```python
from build123d import *

# Parameters (mm, degrees)
SKETCH1_R           = 45
BOSS_EXTRUDE1_DEPTH = 600
SKETCH2_R           = 38.423285368
CUT_EXTRUDE1_DEPTH  = 604.365560834
CHAMFER1_SIZE       = 5.219704
CHAMFER1_SIZE_2     = 9.040792


with BuildPart() as part:
    # Sketch1 → Boss-Extrude1 (new body)
    with BuildSketch(Plane(origin=(0, 0, 0), x_dir=(1, 0, 0), z_dir=(0, 1, 0))):
        with Locations(Location((0, 0, 0), (0, 0, 270))):
            Circle(SKETCH1_R)
    extrude(amount=BOSS_EXTRUDE1_DEPTH)

    # Sketch2 → Cut-Extrude1 (cut, through all)
    with BuildSketch(Plane(origin=(0, 0, 0), x_dir=(1, 0, 0), z_dir=(0, 1, 0))):
        with Locations(Location((0, 0, 0), (0, 0, 270))):
            Circle(SKETCH2_R)
    extrude(amount=CUT_EXTRUDE1_DEPTH, mode=Mode.SUBTRACT)

    # Chamfer1
    # the kernel refuses this chamfer: 9.040792, 5.219704 mm, written as the material it takes off along each edge
    with BuildSketch(Plane(origin=(0, 600, 0), x_dir=(0, 0, 1), z_dir=(-1, 0, 0))) as chamfer1_piece_1:
        Polygon((45, -CHAMFER1_SIZE), (45 - CHAMFER1_SIZE_2, 0), (45, 0), align=None)
    revolve(axis=Axis((0, 600, 0), (0, 1, 0)), mode=Mode.SUBTRACT)
    with BuildSketch(Plane(origin=(0, 0, 0), x_dir=(0, 0, 1), z_dir=(-1, 0, 0))) as chamfer1_piece_2:
        Polygon((45, CHAMFER1_SIZE_2), (45 - CHAMFER1_SIZE, 0), (45, 0), align=None)
    revolve(axis=Axis((0, 0, 0), (0, 1, 0)), mode=Mode.SUBTRACT)


solid = part.part
```
The listing builds one solid part. Answer for the finished solid, in the listing's coordinates (mm). Round coordinates to 2 decimals unless told otherwise and drop trailing zeros. Order: outer loops, then holes, each group sorted by start corner. A loop starts at its lowest first (then second) coordinate and runs counter-clockwise, first axis right, second up. Notation, with made-up numbers: (19.5, 27.5) -> (46.5, 27.5) arc R19 ccw to (46.5, 55.5) -> close; hole circle Ø8 at (-1, 30). An arc over 180 degrees is marked (long way). Answer as CSV lines item,"result".
Q1. A cutting plane is placed at B-B on z = 0. Determine the outline of the cut face in (x, y), plus the area to 3 significant figures.
Computed values:
outline,"(-45, 9.04) -> (-39.78, 0) -> (-38.42, 0) -> (-38.42, 598.58) -> (-45, 594.78) -> close; (38.42, 0) -> (39.78, 0) -> (45, 9.04) -> (45, 594.78) -> (38.42, 598.58) -> close"
area,"7,800 mm^2"
Q2. For a pull along X with two mould halves and no side action, classify faces 1 (the cylindrical face through (-17.235, 297.81, 41.569)), 2 (the flat face through (33, 0, -21)), 3 (the cylindrical face through (11.54, 295.1, 36.65)) as +X half, -X half, draft (parallel to the pull), parting line (faces both ways), or undercut.
Computed values:
face 1,"parting line"
face 2,"draft"
face 3,"undercut"
Q3. Given pin 1 (8 mm diameter, centred on x = 23.5, y = 295, fed in from +Z); pin 2 (1 mm diameter, centred on y = 482, z = 1, fed in from +X); pin 3 (1 mm diameter, centred on y = 327.5, z = -21.5, fed in from +X), each flat-ended and moving along its own axis, determine where each tip first touches the part or whether it passes through.
Computed values:
pin 1,"stops at z = 40.56"
pin 2,"stops at x = 45"
pin 3,"stops at x = 39.8"
Q4. Consider line 1 (X direction, y = 394.5, z = 0); line 2 (X direction, y = 390.5, z = -7); line 3 (Z direction, x = -4, y = 457). Determine where each line is inside the solid, lowest interval first. Write a range as from..to.
Computed values:
line 1,"x = -45..-38.42, 38.42..45"
line 2,"x = -44.45..-37.78, 37.78..44.45"
line 3,"z = -44.82..-38.21, 38.21..44.82"
Q5. A cutting plane is placed at C-C on y = 75. Determine the outline of the cut face in (x, z).
Computed values:
outline,"circle Ø90 at (0, 0); hole circle Ø76.85 at (0, 0)"
Q6. A cutting plane is placed at A-A on x = 0. Determine the outline of the cut face in (y, z), plus the area to 3 significant figures.
Computed values:
outline,"(0, -39.78) -> (9.04, -45) -> (594.78, -45) -> (598.58, -38.42) -> (0, -38.42) -> close; (0, 38.42) -> (598.58, 38.42) -> (594.78, 45) -> (9.04, 45) -> (0, 39.78) -> close"
area,"7,800 mm^2"
